from build123d import *

# Parameters (mm, degrees)
REVOLVE1_ANGLE     = 180
SKETCH2_R          = 1.55
CUT_EXTRUDE1_DEPTH = 9.660254038
SKETCH3_R          = 2.5
CUT_EXTRUDE2_DEPTH = 0.8
CUT_EXTRUDE2_DRAFT = -40


with BuildPart() as part:
    # Sketch1 → Revolve1 (revolve)
    with BuildSketch(Plane(origin=(0, 0, 0), x_dir=(1, 0, 0), z_dir=(0, 1, 0))):
        with BuildLine():
            Line((5, 0), (-5, 0))
            ThreePointArc((-5, 0), (0, 5), (5, 0))
        make_face()
    revolve(axis=Axis((5, 0, 0), (-1, 0, 0)), revolution_arc=REVOLVE1_ANGLE)

    # Sketch2 → Cut-Extrude1 (cut, through all)
    with BuildSketch(Plane(origin=(0, 0, 0), x_dir=(1, 0, 0), z_dir=(0, 1, 0))):
        with Locations(Location((0, 0, 0), (0, 0, 270))):
            Circle(SKETCH2_R)
    extrude(amount=-CUT_EXTRUDE1_DEPTH, mode=Mode.SUBTRACT)


with BuildPart() as cut_extrude2_tool:
    # Sketch3 → Cut-Extrude2 (with draft: the straight prism first)
    with BuildSketch(Plane(origin=(0, 0, 0), x_dir=(1, 0, 0), z_dir=(0, 1, 0))):
        Circle(SKETCH3_R)
    extrude(amount=-CUT_EXTRUDE2_DEPTH)
    # Cut-Extrude2: the draft: its side faces are tilted about the plane it starts from
    cut_extrude2_sides = [cut_extrude2_tool.faces().sort_by_distance(p)[0] for p in [
        (-2.5, -0.4, 0),
    ]]
    draft(cut_extrude2_sides, Plane(origin=(0, 0, 0), x_dir=(1, 0, 0), z_dir=(0, 1, 0)), CUT_EXTRUDE2_DRAFT)


with BuildPart() as part_1:
    add(part.part)

    # Cut-Extrude2: cut by cut_extrude2_tool
    add(cut_extrude2_tool.part, mode=Mode.SUBTRACT)


solid = part_1.part
CAD build for the part. Positions are in the model's coordinates, mm. Give positions to 0.01 mm unless a question says otherwise; leave off trailing zeros. Write each loop counter-clockwise with the first axis right and the second up, starting at its lowest first coordinate (ties: lowest second). Pieces come first, ordered by that corner, then holes. Notation, with made-up numbers: M -36,31.5 L 7,31.5 A7 cw 7,43.5 Z; hole C 37,22 d11. An arc over 180 degrees is marked long. Put each result on its own line as item: value. Start each with the question number.
(1) Band-saw the part on B-B, the plane x = 0. Write the cut outline in (y, z).
(2) Band-saw the part on C-C, the plane y = -1.4. Write the cut outline in (x, z), and give its area (3 significant figures).
(3) Probe L1, parallel to X at y = -2.25, z = 0; L2, parallel to Z at x = 0, y = -3.2; L3, parallel to X at y = -0.9, z = 0.75. List the from-to ranges inside material, lowest first.
(4) Flat gauge pins, fed straight in: pin 1 Ø1 at (x, y) = (-3, -3) entering from +Z; pin 2 Ø1.8 at (x, z) = (0, 0.5) entering from +Y; pin 3 Ø1 at (y, z) = (-0.5, -1) entering from +X; pin 4 Ø1 at (x, z) = (0, -3) entering from -Y. Where does each tip first touch, or does it go through?
(5) Band-saw the part on D-D, the plane z = -3.5. Write the cut outline in (x, y).
(6) Mould opens along Z. For faces 1 (the face through (-2, 0, 2)), 2 (the face through (0.466, -2.749, 1.478)) say: +Z half, -Z half, draft (parallel to the pull), parting line (faces both ways), or undercut.
(7) Band-saw the part on A-A, the plane z = 0. Write the cut outline in (x, y), and give its area (3 significant figures).
Response values:
1. outline: M -4.75,-1.55 A5 ccw 0,-5 L 0,-2.5 L -0.8,-1.83 L -0.8,-1.55 Z; M -4.75,1.55 L -0.8,1.55 L -0.8,1.83 L 0,2.5 L 0,5 A5 ccw Z
2. outline: C 0,0 d9.6; hole C 0,0 d3.1
2. area: 64.8 mm2
3. L1: x = -4.47 to -1.55, 1.55 to 4.47
3. L2: z = -3.84 to -1.55, 1.55 to 3.84
3. L3: x = -4.86 to -1.36, 1.36 to 4.86
4. pin 1: stops at z = 3.32
4. pin 2: passes through
4. pin 3: stops at x = 4.96
4. pin 4: stops at y = -4.33
5. outline: M -3.57,0 A3.57 ccw 3.57,0 Z
6. face 1: draft
6. face 2: undercut
7. outline: M -5,0 A5 ccw -1.55,-4.75 L -1.55,-0.8 L -1.83,-0.8 L -2.5,0 Z; M 1.55,-4.75 A5 ccw 5,0 L 2.5,0 L 1.83,-0.8 L 1.55,-0.8 Z
7. area: 23.0 mm2
